Part model, mm, in its own coordinate system. Face numbers are marked on the shaded views. A direction names the side the tool comes from. Give positions to 0.01 mm unless a question says otherwise; leave off trailing zeros. Write each loop counter-clockwise with the first axis right and the second up, starting at its lowest first coordinate (ties: lowest second). Pieces come first, ordered by that corner, then holes. Notation, with made-up numbers: M 76.25,-26 L 115.25,-26 A13 cw 115.25,-7 Z; hole C 8.25,68 d6. An arc over 180 degrees is marked long. Answer as CSV lines item,"result". Start each with the question number.
1) Tool access for the marked faces 1, 2, 3, 4 and 5: list every direction of +Z, -Z, +X, -X, +Y, -Y with a clear straight run to the whole face (end or side of a thin tool).
2) Pin check, flat tips, straight feed: pin 1 Ø1.5 at (x, z) = (20.5, 2.5) entering from -Y; pin 2 Ø1 at (x, z) = (28, 1) entering from -Y. Stop position of each tip, or through.
3) Mould opens along X. For the marked faces 6, 7, 8 and 9 say: pulls with the +X half, pulls with the -X half, needs draft (parallel to the pull), parting line crosses it, or undercut.
4) Slice it at B-B, the plane x = 23.5. Give the cut face in (y, z), plus the area to 3 significant figures.
5) Wall check: line 1 along Y through (x, z) = (0, 1.1); line 2 along X through (y, z) = (13.75, 3.25); line 3 along Y through (x, z) = (18, 0.4). Give the ranges that are in metal, low to high. Write a range as from..to.
6) Slice it at A-A, the plane z = 1.95. Give the number of separate pieces and of enclosed holes in the cut face, plus the area to 3 significant figures.
```python
from build123d import *

# Parameters (mm, degrees)
SKETCH1_R           = 1.75
BOSS_EXTRUDE1_DEPTH = 4
SKETCH2_R           = 1.75
CUT_EXTRUDE2_DEPTH  = 38.915688046
SKETCH3_R           = 2.4
SKETCH3_R_2         = 1.3
CUT_EXTRUDE3_DEPTH  = 38.915688046


with BuildPart() as part:
    # Sketch1 → Boss-Extrude1 (new body)
    with BuildSketch(Plane.XY):
        with BuildLine():
            Line((0.31, 14.63), (-0.31, 14.63))
            ThreePointArc((-0.31, 14.63), (-0.838273314, 13.383704325), (-1.04, 12.04518576))
            ThreePointArc((-1.04, 12.04518576), (-1.578061664, 11.986568374), (-2.112960617, 11.903927815))
            ThreePointArc((-2.112960617, 11.903927815), (-2.65424773, 13.144626757), (-3.487085624, 14.211728743))
            Line((-3.487085624, 14.211728743), (-4.085959636, 14.051260935))
            ThreePointArc((-4.085959636, 14.051260935), (-4.273667417, 12.71070456), (-4.122086336, 11.365584201))
            ThreePointArc((-4.122086336, 11.365584201), (-4.626642697, 11.169703548), (-5.12192646, 10.951436862))
            ThreePointArc((-5.12192646, 10.951436862), (-5.965886177, 12.009764599), (-7.046532125, 12.824951657))
            Line((-7.046532125, 12.824951657), (-7.583467875, 12.514951657))
            ThreePointArc((-7.583467875, 12.514951657), (-7.417818147, 11.171491285), (-6.9232593, 9.911436862))
            ThreePointArc((-6.9232593, 9.911436862), (-7.359925677, 9.591641884), (-7.781841479, 9.252623584))
            ThreePointArc((-7.781841479, 9.252623584), (-8.870959341, 10.05645683), (-10.125769107, 10.564175311))
            Line((-10.125769107, 10.564175311), (-10.564175311, 10.125769107))
            ThreePointArc((-10.564175311, 10.125769107), (-10.05645683, 8.870959341), (-9.252623584, 7.781841479))
            ThreePointArc((-9.252623584, 7.781841479), (-9.591641884, 7.359925677), (-9.911436862, 6.9232593))
            ThreePointArc((-9.911436862, 6.9232593), (-11.171491285, 7.417818147), (-12.514951657, 7.583467875))
            Line((-12.514951657, 7.583467875), (-12.824951657, 7.046532125))
            ThreePointArc((-12.824951657, 7.046532125), (-12.009764599, 5.965886177), (-10.951436862, 5.12192646))
            ThreePointArc((-10.951436862, 5.12192646), (-11.169703548, 4.626642697), (-11.365584201, 4.122086336))
            ThreePointArc((-11.365584201, 4.122086336), (-12.71070456, 4.273667417), (-14.051260935, 4.085959636))
            Line((-14.051260935, 4.085959636), (-14.211728743, 3.487085624))
            ThreePointArc((-14.211728743, 3.487085624), (-13.144626757, 2.65424773), (-11.903927815, 2.112960617))
            ThreePointArc((-11.903927815, 2.112960617), (-11.986568374, 1.578061664), (-12.04518576, 1.04))
            ThreePointArc((-12.04518576, 1.04), (-13.383704325, 0.838273314), (-14.63, 0.31))
            Line((-14.63, 0.31), (-14.63, -0.31))
            ThreePointArc((-14.63, -0.31), (-13.383704325, -0.838273314), (-12.04518576, -1.04))
            ThreePointArc((-12.04518576, -1.04), (-11.986568374, -1.578061664), (-11.903927815, -2.112960617))
            ThreePointArc((-11.903927815, -2.112960617), (-13.144626757, -2.65424773), (-14.211728743, -3.487085624))
            Line((-14.211728743, -3.487085624), (-14.051260935, -4.085959636))
            ThreePointArc((-14.051260935, -4.085959636), (-12.71070456, -4.273667417), (-11.365584201, -4.122086336))
            ThreePointArc((-11.365584201, -4.122086336), (-11.169703548, -4.626642697), (-10.951436862, -5.12192646))
            ThreePointArc((-10.951436862, -5.12192646), (-12.009764599, -5.965886177), (-12.824951657, -7.046532125))
            Line((-12.824951657, -7.046532125), (-12.514951657, -7.583467875))
            ThreePointArc((-12.514951657, -7.583467875), (-11.171491285, -7.417818147), (-9.911436862, -6.9232593))
            ThreePointArc((-9.911436862, -6.9232593), (1.578061664, -11.986568374), (11.365584201, -4.122086336))
            Line((11.365584201, -4.122086336), (30.75, -4))
            ThreePointArc((30.75, -4), (34.75, 0), (30.75, 4))
            Line((30.75, 4), (11.365584201, 4.122086336))
            ThreePointArc((11.365584201, 4.122086336), (11.169703548, 4.626642697), (10.951436862, 5.12192646))
            ThreePointArc((10.951436862, 5.12192646), (12.009764599, 5.965886177), (12.824951657, 7.046532125))
            Line((12.824951657, 7.046532125), (12.514951657, 7.583467875))
            ThreePointArc((12.514951657, 7.583467875), (11.171491285, 7.417818147), (9.911436862, 6.9232593))
            ThreePointArc((9.911436862, 6.9232593), (9.591641884, 7.359925677), (9.252623584, 7.781841479))
            ThreePointArc((9.252623584, 7.781841479), (10.05645683, 8.870959341), (10.564175311, 10.125769107))
            Line((10.564175311, 10.125769107), (10.125769107, 10.564175311))
            ThreePointArc((10.125769107, 10.564175311), (8.870959341, 10.05645683), (7.781841479, 9.252623584))
            ThreePointArc((7.781841479, 9.252623584), (7.359925677, 9.591641884), (6.9232593, 9.911436862))
            ThreePointArc((6.9232593, 9.911436862), (7.417818147, 11.171491285), (7.583467875, 12.514951657))
            Line((7.583467875, 12.514951657), (7.046532125, 12.824951657))
            ThreePointArc((7.046532125, 12.824951657), (5.965886177, 12.009764599), (5.12192646, 10.951436862))
            ThreePointArc((5.12192646, 10.951436862), (4.626642697, 11.169703548), (4.122086336, 11.365584201))
            ThreePointArc((4.122086336, 11.365584201), (4.273667417, 12.71070456), (4.085959636, 14.051260935))
            Line((4.085959636, 14.051260935), (3.487085624, 14.211728743))
            ThreePointArc((3.487085624, 14.211728743), (2.65424773, 13.144626757), (2.112960617, 11.903927815))
            ThreePointArc((2.112960617, 11.903927815), (1.578061664, 11.986568374), (1.04, 12.04518576))
            ThreePointArc((1.04, 12.04518576), (0.838273314, 13.383704325), (0.31, 14.63))
        make_face()
        with Locations((30.75, 0)):
            Circle(SKETCH1_R, mode=Mode.SUBTRACT)
    extrude(amount=BOSS_EXTRUDE1_DEPTH)

    # Sketch2 → Cut-Extrude2 (cut, through all)
    with BuildSketch(Plane.XY.offset(4)):
        Circle(SKETCH2_R)
    extrude(amount=-CUT_EXTRUDE2_DEPTH, mode=Mode.SUBTRACT)

    # Sketch3 → Cut-Extrude3 (cut, through all)
    with BuildSketch(Plane.XY.offset(4)):
        Circle(SKETCH3_R)
        with Locations((-4.5, 0)):
            Circle(SKETCH3_R_2)
        with Locations((4.5, 0)):
            Circle(SKETCH3_R_2)
    extrude(amount=-CUT_EXTRUDE3_DEPTH, mode=Mode.SUBTRACT)


solid = part.part
```
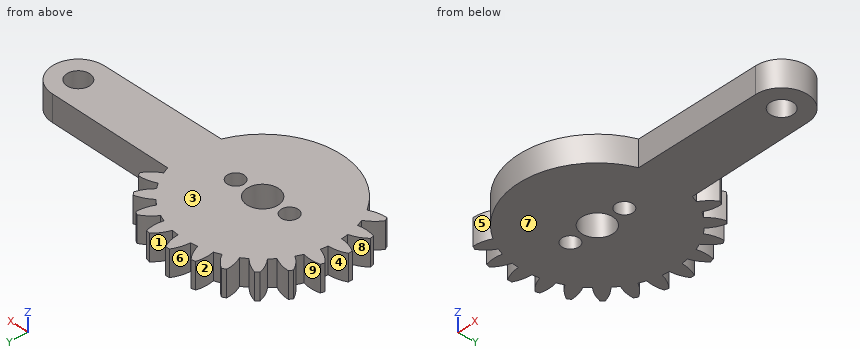
Found:
1,face 1,"+Z, -Z, +Y"
1,face 2,"+Z, -Z"
1,face 3,"+Z, +X, -X, +Y, -Y"
1,face 4,"+Z, -Z, -X"
1,face 5,"+Z, -Z, -Y"
2,pin 1,"y = -4.07"
2,pin 2,"y = -4.02"
3,face 6,"undercut"
3,face 7,"needs draft"
3,face 8,"pulls with the -X half"
3,face 9,"undercut"
4,outline,"M -4.05,0 L 4.05,0 L 4.05,4 L -4.05,4 Z"
4,area,"32.4 mm²"
5,line 1,"-12.09..-2.4, 2.4..14.63"
5,line 2,"-4.16..-3.07, -0.72..0.72, 3.07..4.16"
5,line 3,"-4.08..4.08"
6,separate pieces,"1"
6,enclosed holes,"4"
6,area,"652 mm²"
